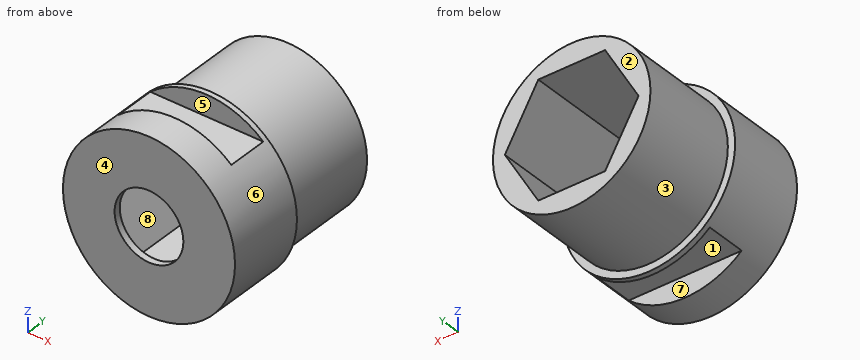
from build123d import *

# Parameters (mm, degrees)
SKETCH1_R               = 7.5565
BOSS_EXTRUDE1_DEPTH     = 16.51
SKETCH2_R               = 7.5565
SKETCH2_R_2             = 3.3
BOSS_EXTRUDE2_DEPTH     = 0.635
SKETCH4_R               = 8.255
SKETCH4_R_2             = 7.5565
BOSS_EXTRUDE3_DEPTH     = 7.62
SKETCH3_W               = 2.572814656
SKETCH3_H               = 3.937
SKETCH3_W_2             = 2.256055482
CUT_EXTRUDE1_DEPTH      = 9.255
CUT_EXTRUDE1_DEPTH_BACK = 9.255


with BuildPart() as part:
    # Sketch1 → Boss-Extrude1 (new body)
    with BuildSketch(Plane(origin=(0, 0, 0), x_dir=(1, 0, 0), z_dir=(0, 1, 0))):
        Circle(SKETCH1_R)
        Polygon((-3.207902433, 5.55625), (-6.415804866, 0), (-3.207902433, -5.55625), (3.207902433, -5.55625), (6.415804866, 0), (3.207902433, 5.55625), align=None, mode=Mode.SUBTRACT)
    extrude(amount=BOSS_EXTRUDE1_DEPTH)

    # Sketch2 → Boss-Extrude2 (add)
    with BuildSketch(Plane.XZ):
        Circle(SKETCH2_R)
        Circle(SKETCH2_R_2, mode=Mode.SUBTRACT)
    extrude(amount=BOSS_EXTRUDE2_DEPTH)

    # Sketch4 → Boss-Extrude3 (add)
    with BuildSketch(Plane.XZ.offset(0.635)):
        Circle(SKETCH4_R)
        Circle(SKETCH4_R_2, mode=Mode.SUBTRACT)
    extrude(amount=-BOSS_EXTRUDE3_DEPTH)

    # Sketch3 → Cut-Extrude1 (cut, two sides)
    with BuildSketch(Plane(origin=(0, 0, 0), x_dir=(0, 0, -1), z_dir=(1, 0, 0))) as cut_extrude1_sk:
        with Locations((-7.509407328, 4.5085)):
            Rectangle(SKETCH3_W, SKETCH3_H)
        with Locations((7.351027741, 4.5085)):
            Rectangle(SKETCH3_W_2, SKETCH3_H)
    extrude(amount=CUT_EXTRUDE1_DEPTH, mode=Mode.SUBTRACT)
    extrude(cut_extrude1_sk.sketch, amount=-CUT_EXTRUDE1_DEPTH_BACK, mode=Mode.SUBTRACT)


solid = part.part
Here's how the part is built. I have some questions about the finished solid (model axes, mm). Face numbers are marked on the shaded views. A direction names the side the tool comes from. Round coordinates to 2 decimals unless told otherwise and drop trailing zeros. Write each loop counter-clockwise with the first axis right and the second up, starting at its lowest first coordinate (ties: lowest second). Pieces come first, ordered by that corner, then holes.
1. If we mould it in two halves opening along Z, with no side actions, what happens to the marked faces 6, 7 and 8? For each: released by +Z, released by -Z, zero draft, split by the parting line, or undercut.
2. Suppose I cut it at A-A (y = 1.5). List the corners of the cut face in (x, z) for me (3 decimals), and give its area (3 significant figures).
3. Suppose I cut it at D-D (z = -5). List the corners of the cut face in (x, y) for me (3 decimals), and give its area (3 significant figures).
4. Suppose I cut it at C-C (z = -2.5). List the corners of the cut face in (x, y) for me (3 decimals).
5. Suppose I cut it at B-B (x = 0). List the corners of the cut face in (y, z) for me (1 decimal), and give its area (3 significant figures).
6. For the marked faces 1, 2, 3, 4 and 5, which set-ups out of +Z, -Z, +X, -X, +Y, -Y let a thin tool reach every point of the face, with its end or its side?
7. I need wall thicknesses on L1, parallel to Z at x = -0.5, y = 3; L2, parallel to Z at x = 0, y = -0.35 (3 decimals); L3, parallel to Y at x = -2.25, z = -6.5 (3 decimals). Which ranges of each line are inside material? Lowest first, please.
8. Will these pins go through, and if not, where does the flat tip stop? pin 1 Ø1.2 at (x, y) = (2.5, 4) entering from +Z; pin 2 Ø2 at (x, y) = (0.5, 4.5) entering from -Z.
Answer sheet:
1. face 6: split by the parting line
1. face 7: zero draft
1. face 8: undercut
2. outline: circle Ø16.51 at (0, 0); hole (-6.416, 0) - (-3.208, -5.556) - (3.208, -5.556) - (6.416, 0) - (3.208, 5.556) - (-3.208, 5.556) - close
2. area: 107 mm2
3. outline: (-6.568, -0.635) - (6.568, -0.635) - (6.568, 6.985) - (5.666, 6.985) - (5.666, 16.51) - (3.529, 16.51) - (3.529, 0) - (-3.529, 0) - (-3.529, 16.51) - (-5.666, 16.51) - (-5.666, 6.985) - (-6.568, 6.985) - close
3. area: 91.5 mm2
4. outline: (-7.867, -0.635) - (-2.154, -0.635) - (-2.154, 0) - (-4.972, 0) - (-4.972, 16.51) - (-7.131, 16.51) - (-7.131, 6.985) - (-7.867, 6.985) - close; (2.154, -0.635) - (7.867, -0.635) - (7.867, 6.985) - (7.131, 6.985) - (7.131, 16.51) - (4.972, 16.51) - (4.972, 0) - (2.154, 0) - close
5. outline: (-0.6, -8.3) - (2.5, -8.3) - (2.5, -6.2) - (6.5, -6.2) - (6.5, -8.3) - (7, -8.3) - (7, -7.6) - (16.5, -7.6) - (16.5, -5.6) - (0, -5.6) - (0, -3.3) - (-0.6, -3.3) - close; (-0.6, 3.3) - (0, 3.3) - (0, 5.6) - (16.5, 5.6) - (16.5, 7.6) - (7, 7.6) - (7, 8.3) - (6.5, 8.3) - (6.5, 6.2) - (2.5, 6.2) - (2.5, 8.3) - (-0.6, 8.3) - close
5. area: 66.1 mm2
6. face 1: -Z, +X, -X
6. face 2: +Z, -Z, +X, -X, +Y
6. face 3: +Y
6. face 4: +Z, -Z, +X, -X, -Y
6. face 5: +Z, +X, -X
7. L1: z = -6.22 to -5.56, 5.56 to 6.22
7. L2: z = -8.255 to -3.3, 3.3 to 8.255
7. L3: y = -0.635 to 2.54, 6.477 to 16.51
8. pin 1: stops at z = 6.22
8. pin 2: stops at z = -6.22
